Source: CAD feature listing. Evaluate the final solid. Frame: model axes, mm. Face numbers are marked on the shaded views. A direction names the side the tool comes from. Give positions to 0.01 mm unless a question says otherwise; leave off trailing zeros. Write each loop counter-clockwise with the first axis right and the second up, starting at its lowest first coordinate (ties: lowest second). Pieces come first, ordered by that corner, then holes. Notation, with made-up numbers: M 75.25,82 L 79.25,82 A18 ccw 79.25,110 Z; hole C -38.75,35 d10. An arc over 180 degrees is marked long. Use CSV: the item, a comma, the result in double quotes. Start each with the question number.
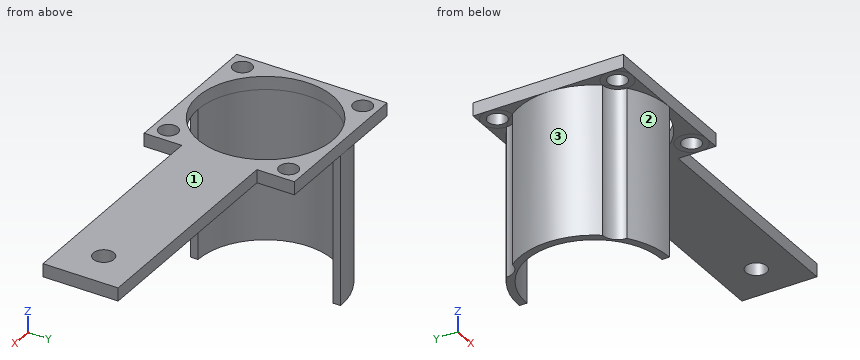
from build123d import *

# Parameters (mm, degrees)
F0_W     = 40
F0_H     = 40
F0_R     = 2.5
F0_R_2   = 18
F1_DEPTH = 3.5
F2_W     = 60
F2_H     = 20
F2_R     = 2.75
F3_DEPTH = 3.5
F7_DEPTH = 40
F8_R     = 4
F9_DEPTH = 40.001


with BuildPart() as f1:
    # F0 (on Top) → F1 (new body)
    with BuildSketch(Plane.XY):
        with Locations((20, 20)):
            Rectangle(F0_W, F0_H)
        with Locations((4, 4)):
            Circle(F0_R, mode=Mode.SUBTRACT)
        with Locations((36, 4)):
            Circle(F0_R, mode=Mode.SUBTRACT)
        with Locations((4, 36)):
            Circle(F0_R, mode=Mode.SUBTRACT)
        with Locations((20, 20)):
            Circle(F0_R_2, mode=Mode.SUBTRACT)
        with Locations((36, 36)):
            Circle(F0_R, mode=Mode.SUBTRACT)
    extrude(amount=F1_DEPTH)

    # F2 (on face) → F3 (join, through all)
    with BuildSketch(Plane.XY.offset(3.5)):
        with Locations((70, 20)):
            Rectangle(F2_W, F2_H)
        with Locations((90, 20)):
            Circle(F2_R, mode=Mode.SUBTRACT)
    extrude(amount=-F3_DEPTH)

    # F6 (on face) → F7 (join, through all)
    with BuildSketch(Plane.XY):
        with BuildLine():
            Line((20, 38), (20, 40))
            ThreePointArc((20, 40), (0, 20), (20, 0))
            Line((20, 0), (20, 2))
            ThreePointArc((20, 2), (2, 20), (20, 38))
        make_face()
    extrude(amount=-F7_DEPTH)

    # F8 (on face) → F9 (cut, through all)
    with BuildSketch(Plane.XY):
        with Locations((36, 36)):
            Circle(F8_R)
        with Locations((4, 36)):
            Circle(F8_R)
        with Locations((4, 4)):
            Circle(F8_R)
        with Locations((36, 4)):
            Circle(F8_R)
    extrude(amount=-F9_DEPTH, mode=Mode.SUBTRACT)


solid = f1.part
Item 1: Section C-C (y = 15). Return the cut outline in (x, z), plus the area to 3 significant figures.
Item 2: Section A-A (x = 90). Return the cut outline in (y, z), plus the area to 4 significant figures.
Item 3: Contact query for flat-ended pins moving along their axis: pin 1 Ø10 at (x, z) = (80.5, -9.5) entering from +Y; pin 2 Ø3 at (y, z) = (34, 2.5) entering from +X; pin 3 Ø12 at (x, y) = (36, 18) entering from +Z; pin 4 Ø4 at (x, z) = (66, 1.5) entering from +Y. Output: stop coordinate, or through.
Item 4: Material intervals for probe 1 along Y at (x, z) = (90, 1); probe 2 along Y at (x, z) = (4, 2.75); probe 3 along Z at (x, y) = (30, 35), sorted ascending.
Item 5: Set-up query: the marked faces 1, 2 and 3. Return all of +Z, -Z, +X, -X, +Y, -Y with unobstructed straight access to the full face (end or side cutting, diameter ignored); none if empty.
Item 6: Section D-D (y = 34.5). Return the cut outline in (x, z), plus the area to 3 significant figures.
Item 7: Section B-B (z = -6). Return the cut outline in (x, y).
Output values:
1,outline,"M 0,0 L 0.64,0 L 0.64,-40 L 2.71,-40 L 2.71,3.5 L 0,3.5 Z; M 37.29,0 L 100,0 L 100,3.5 L 37.29,3.5 Z"
1,area,"312 mm2"
2,outline,"M 10,0 L 17.25,0 L 17.25,3.5 L 10,3.5 Z; M 22.75,0 L 30,0 L 30,3.5 L 22.75,3.5 Z"
2,area,"50.75 mm2"
3,pin 1,"passes through"
3,pin 2,"stops at x = 40"
3,pin 3,"stops at z = 3.5"
3,pin 4,"stops at y = 30"
4,probe 1,"y = 10 to 17.25, 22.75 to 30"
4,probe 2,"y = 0 to 1.5, 6.5 to 11.75, 28.25 to 33.5, 38.5 to 40"
4,probe 3,"z = 0 to 3.5"
5,face 1,"+Z, +X, -X, +Y, -Y"
5,face 2,"-Z, -X, -Y"
5,face 3,"-Z, -X"
6,outline,"M 0,0 L 2,0 L 2,3.5 L 0,3.5 Z; M 6,0 L 7.71,0 L 7.71,-40 L 9.33,-40 L 9.33,3.5 L 6,3.5 Z; M 30.67,0 L 34,0 L 34,3.5 L 30.67,3.5 Z; M 38,0 L 40,0 L 40,3.5 L 38,3.5 Z"
6,area,"102 mm2"
7,outline,"M 4,8 A4 cw 8,4 A20 ccw 20,0 L 20,2 A18 cw 20,38 L 20,40 A20 ccw 8,36 A4 cw 4,32 A20 ccw Z"
